Geometry check sheet. Reference: the model listing, model coordinates, mm. A direction names the side the tool comes from. Coordinates: 2 decimals unless noted, no trailing zeros. Loops run counter-clockwise (first coordinate to the right, second up) from the corner with the lowest first, then second, coordinate; pieces in that order, holes last. Notation, with made-up numbers: (-2.5, -18) -> (33.5, -18) arc R23 cw to (33.5, 9) -> close; hole circle Ø1 at (60, -34). An arc over 180 degrees is marked (long way). Answer as a JSON object with one key per item and string values.
from build123d import *

# Parameters (mm, degrees)
SKETCH1_W           = 52.2
SKETCH1_H           = 28.5
SKETCH1_R           = 1
SKETCH1_W_2         = 35.320636832
SKETCH1_H_2         = 5.8
BOSS_EXTRUDE1_DEPTH = 2.5
FILLET1_R           = 2
FILLET2_R           = 2.9
SKETCH4_R           = 2
CUT_EXTRUDE1_DEPTH  = 1.4


with BuildPart() as part:
    # Sketch1 → Boss-Extrude1 (new body)
    with BuildSketch(Plane(origin=(0, 0, 0), x_dir=(1, 0, 0), z_dir=(0, 1, 0))):
        with Locations((0, 2.55)):
            Rectangle(SKETCH1_W, SKETCH1_H)
        with Locations(Location((-22.8, -3.2, 0), (0, 0, 270))):
            Circle(SKETCH1_R, mode=Mode.SUBTRACT)
        with Locations(Location((22.8, -3.2, 0), (0, 0, 90))):
            Circle(SKETCH1_R, mode=Mode.SUBTRACT)
        with Locations(Location((22.8, 8.3, 0), (0, 0, 270))):
            Circle(SKETCH1_R, mode=Mode.SUBTRACT)
        with Locations(Location((-22.8, 8.3, 0), (0, 0, 90))):
            Circle(SKETCH1_R, mode=Mode.SUBTRACT)
        with Locations((0, -4.8)):
            Rectangle(SKETCH1_W_2, SKETCH1_H_2, mode=Mode.SUBTRACT)
        with Locations((0, 9.9)):
            Rectangle(SKETCH1_W_2, SKETCH1_H_2, mode=Mode.SUBTRACT)
    extrude(amount=BOSS_EXTRUDE1_DEPTH)

    # Fillet1
    fillet1_edges = [part.edges().sort_by_distance(p)[0] for p in [
        (26.1, 1.25, 11.7),
        (-26.1, 1.25, 11.7),
        (-26.1, 1.25, -16.8),
        (26.1, 1.25, -16.8),
    ]]
    fillet(fillet1_edges, radius=FILLET1_R)

    # Fillet2
    fillet2_edges = [part.edges().sort_by_distance(p)[0] for p in [
        (17.660318416, 1.25, -7),
        (17.660318416, 1.25, -12.8),
        (17.660318416, 1.25, 7.7),
        (17.660318416, 1.25, 1.9),
        (-17.660318416, 1.25, 7.7),
        (-17.660318416, 1.25, 1.9),
        (-17.660318416, 1.25, -7),
        (-17.660318416, 1.25, -12.8),
    ]]
    fillet(fillet2_edges, radius=FILLET2_R - 0.0001)  # a hair under: the kernel refuses the full size

    # Sketch4 → Cut-Extrude1 (cut)
    with BuildSketch(Plane(origin=(0, 2.5, 0), x_dir=(1, 0, 0), z_dir=(0, 1, 0))):
        with Locations(Location((-22.8, 8.3, 0), (0, 0, 270))):
            Circle(SKETCH4_R)
        with Locations(Location((-22.8, -3.2, 0), (0, 0, 270))):
            Circle(SKETCH4_R)
        with Locations(Location((22.8, -3.2, 0), (0, 0, 270))):
            Circle(SKETCH4_R)
        with Locations(Location((22.8, 8.3, 0), (0, 0, 270))):
            Circle(SKETCH4_R)
    extrude(amount=-CUT_EXTRUDE1_DEPTH, mode=Mode.SUBTRACT)


solid = part.part
1. Thickness scan on probe 1 along Z at (x, y) = (15, 1.4); probe 2 along X at (y, z) = (1.9, 3.2); probe 3 along X at (y, z) = (0.7, -8.3). Record the ranges inside material, lowest first. Write a range as from..to.
Evaluation:
{"probe 1": "z = -16.8..-12.79, -7.01..1.91, 7.69..11.7", "probe 2": "x = -26.1..-24.8, -20.8..-17.18, 17.18..20.8, 24.8..26.1", "probe 3": "x = -26.1..-23.8, -21.8..-17.18, 17.18..21.8, 23.8..26.1"}
2. Section check B-B, the plane x = 22.8. Record the boundary of the cut face in (y, z), then the cut area to 4 significant figures.
Evaluation:
{"outline": "(0, -16.8) -> (2.5, -16.8) -> (2.5, -10.3) -> (1.1, -10.3) -> (1.1, -9.3) -> (0, -9.3) -> close; (0, -7.3) -> (1.1, -7.3) -> (1.1, -6.3) -> (2.5, -6.3) -> (2.5, 1.2) -> (1.1, 1.2) -> (1.1, 2.2) -> (0, 2.2) -> close; (0, 4.2) -> (1.1, 4.2) -> (1.1, 5.2) -> (2.5, 5.2) -> (2.5, 11.7) -> (0, 11.7) -> close", "area": "55.65 mm^2"}
3. Mould release check, pull along X, two halves, no side actions. Record for faces 4 (the face through (0, 2.5, -3)), 5 (the face through (-16.79, 1.27, -7.83)), 6 (the face through (-26.1, 1, -2)), 7 (the face through (25.5, 1.27, -16.23)): released by +X, released by -X, zero draft, split by the parting line, or undercut.
Evaluation:
{"face 4": "zero draft", "face 5": "undercut", "face 6": "released by -X", "face 7": "released by +X"}
4. Depth check by flat-ended pin: P1, Ø2.5, axis at x = -22.8, z = 3.2, coming from the +Y side; P2, Ø1.8, axis at x = 22.8, z = 3.2, coming from the +Y side. Enter the tip coordinate at first touch or a pass-through.
Evaluation:
{"P1": "stops at y = 1.1", "P2": "passes through"}
5. Section check C-C, the plane z = 3.2. Record the boundary of the cut face in (x, y).
Evaluation:
{"outline": "(-26.1, 0) -> (-23.8, 0) -> (-23.8, 1.1) -> (-24.8, 1.1) -> (-24.8, 2.5) -> (-26.1, 2.5) -> close; (-21.8, 0) -> (-17.18, 0) -> (-17.18, 2.5) -> (-20.8, 2.5) -> (-20.8, 1.1) -> (-21.8, 1.1) -> close; (17.18, 0) -> (21.8, 0) -> (21.8, 1.1) -> (20.8, 1.1) -> (20.8, 2.5) -> (17.18, 2.5) -> close; (23.8, 0) -> (26.1, 0) -> (26.1, 2.5) -> (24.8, 2.5) -> (24.8, 1.1) -> (23.8, 1.1) -> close"}
6. Section check D-D, the plane x = -3. Record the boundary of the cut face in (y, z), then the cut area to 4 significant figures.
Evaluation:
{"outline": "(0, -16.8) -> (2.5, -16.8) -> (2.5, -12.8) -> (0, -12.8) -> close; (0, -7) -> (2.5, -7) -> (2.5, 1.9) -> (0, 1.9) -> close; (0, 7.7) -> (2.5, 7.7) -> (2.5, 11.7) -> (0, 11.7) -> close", "area": "42.25 mm^2"}
7. Tool access check on faces 1 (the face through (0, 1, -16.8)), 2 (the face through (-24.752, 1.81, 2.766)), 3 (the face through (-16.79, 1.27, 6.87)). Record the directions out of +Z, -Z, +X, -X, +Y, -Y that give a thin tool (end or side, any length) a straight path to the whole face; none if there is none.
Evaluation:
{"face 1": "-Z, +X, -X, +Y, -Y", "face 2": "+Y", "face 3": "+Y, -Y"}
8. Section check A-A, the plane y = 0.4. State how many separate pieces and enclosed holes the cut face has, then the cut area to 3 significant figures.
Evaluation:
{"separate pieces": "1", "enclosed holes": "6", "area": "1,080 mm^2"}
